```python
from build123d import *

# Parameters (mm, degrees)
BOSS_EXTRUDE1_DEPTH = 18
SKETCH3_R           = 2.5
SKETCH3_R_2         = 3
CUT_EXTRUDE1_DEPTH  = 40.102429592


with BuildPart() as part:
    # Sketch1 → Boss-Extrude1 (new body)
    with BuildSketch(Plane(origin=(0, 0, 0), x_dir=(1, 0, 0), z_dir=(0, 1, 0))):
        Polygon((-8.25, 7.5), (-8.25, -23.604773379), (14.75, -7.5), (14.75, 7.5), (4.25, 7.5), (4.25, 26), (-4.25, 26), (-4.25, 7.5), align=None)
    extrude(amount=BOSS_EXTRUDE1_DEPTH)

    # Sketch3 → Cut-Extrude1 (cut, through all)
    with BuildSketch(Plane.ZY.offset(8.25)):
        with Locations((-17, 9)):
            Circle(SKETCH3_R)
        with Locations((-3, 9)):
            Circle(SKETCH3_R_2)
        with Locations((4.5, 9)):
            Circle(SKETCH3_R_2)
        with BuildLine():
            Line((-26, 9), (-26, 18))
            Line((-26, 18), (-17, 18))
            ThreePointArc((-17, 18), (-23.363961031, 15.363961031), (-26, 9))
        make_face()
    extrude(amount=-CUT_EXTRUDE1_DEPTH, mode=Mode.SUBTRACT)


solid = part.part
```
Can you work these out from the model? Positions are in its coordinate system, mm. A direction names the side the tool comes from. Give positions to 0.01 mm unless a question says otherwise; leave off trailing zeros. Loops run counter-clockwise (first coordinate to the right, second up) from the corner with the lowest first, then second, coordinate; pieces in that order, holes last. Notation, with made-up numbers: M 35,34.25 L 53,34.25 A29 cw 53,59.25 Z; hole C 82.25,66.5 d9. An arc over 180 degrees is marked long. One line per item, written item: value.
(1) I need wall thicknesses on line 1 (Z direction, x = 3.25, y = 11); line 2 (Z direction, x = -0.5, y = 10); line 3 (Z direction, x = 7.75, y = 6.5). Which ranges of each line are inside material? Lowest first, please.
Returned:
line 1: -25.77 to -18.5, -15.5 to -5.24, -0.76 to 2.26, 6.74 to 15.55
line 2: -25.94 to -19.29, -14.71 to -5.83, -0.17 to 1.67, 7.33 to 18.18
line 3: -7.5 to -4.66, -1.34 to 2.84, 6.16 to 12.4
(2) Suppose I cut it at A-A on z = -3. List the corners of the cut face in (x, y) for me.
Returned:
outline: M -8.25,0 L 14.75,0 L 14.75,6 L -8.25,6 Z; M -8.25,12 L 14.75,12 L 14.75,18 L -8.25,18 Z
(3) We'd pull the mould along Y, two halves only. Please class faces 1 (the face through (-0.1, 7.5, -19)), 2 (the face through (-0.059, 15.434, -23.294)), 3 (the face through (-4.25, 7, -15)): released by +Y, released by -Y, zero draft, split by the parting line, or undercut.
Returned:
face 1: undercut
face 2: released by +Y
face 3: zero draft
(4) Which directions (+Z, -Z, +X, -X, +Y, -Y) give clear straight access to the entire face, cutting with the end or side of a thin tool? Please do faces 4 (the face through (10, 9, -7.5)), 5 (the face through (-6, 9, -7.5)), 6 (the face through (3.1, 9.1, 1.5)).
Returned:
face 4: -Z, +X, +Y, -Y
face 5: -Z, -X, +Y, -Y
face 6: +X, -X
(5) Will these pins go through, and if not, where does the flat tip stop? pin 1 (8.5 mm diameter, centred on x = 10.5, y = 12.5, fed in from -Z); pin 2 (1 mm diameter, centred on y = 14.5, z = 15.5, fed in from +X); pin 3 (8 mm diameter, centred on x = 1, y = 5, fed in from +Z); pin 4 (3.5 mm diameter, centred on y = 9, z = -3, fed in from +X).
Returned:
pin 1: z = -7.5
pin 2: x = 4.04
pin 3: z = 19.93
pin 4: through
(6) Suppose I cut it at C-C on x = -1.5. List the corners of the cut face in (y, z) for me, plus the area to 3 significant figures.
Returned:
outline: M 0,-26 L 9,-26 A9 ccw 18,-17 L 18,18.88 L 0,18.88 Z; hole C 9,-3 d6; hole C 9,4.5 d6; hole C 9,-17 d5
area: 714 mm^2
(7) Suppose I cut it at D-D on z = -16.5. List the corners of the cut face in (x, y) for me, plus the area to 3 significant figures.
Returned:
outline: M -4.25,0 L 4.25,0 L 4.25,6.55 L -4.25,6.55 Z; M -4.25,11.45 L 4.25,11.45 L 4.25,18 L -4.25,18 Z
area: 111 mm^2
(8) Suppose I cut it at B-B on y = 3.25. List the corners of the cut face in (x, z) for me.
Returned:
outline: M -8.25,-7.5 L -4.25,-7.5 L -4.25,-26 L 4.25,-26 L 4.25,-7.5 L 14.75,-7.5 L 14.75,7.5 L -8.25,23.6 Z
